from build123d import *

# Parameters (mm, degrees)
SKETCH3_W           = 5
SKETCH3_H           = 30
BOSS_EXTRUDE1_DEPTH = 5
SKETCH4_R           = 1.6
CUT_EXTRUDE1_DEPTH  = 75.540257579


with BuildPart() as part:
    # Sketch2 → Revolve1 (revolve)
    with BuildSketch(Plane.XY):
        with BuildLine():
            Line((0, 29), (0, 30))
            ThreePointArc((0, 30), (21.213203436, 21.213203436), (30, 0))
            Line((30, 0), (29, 0))
            ThreePointArc((29, 0), (20.506096654, 20.506096654), (0, 29))
        make_face()
    revolve(axis=Axis((0, 0, 0), (0, 1, 0)))

    # Sketch3 → Boss-Extrude1 (add)
    with BuildSketch(Plane.XZ):
        with Locations((0, -45)):
            Rectangle(SKETCH3_W, SKETCH3_H)
        with BuildLine():
            Line((-2.5, -38), (2.5, -38))
            Line((2.5, -38), (12.22277757, -26.308006594))
            Line((12.22277757, -26.308006594), (12.219091313, -26.300072385))
            ThreePointArc((12.219091313, -26.300072385), (-0.967100454, -29.109666297), (-13.937737405, -25.431073041))
            Line((-13.937737405, -25.431073041), (-14.41834904, -26.308006594))
            Line((-14.41834904, -26.308006594), (-2.5, -38))
        make_face()
    extrude(amount=-BOSS_EXTRUDE1_DEPTH)

    # Sketch4 → Cut-Extrude1 (cut, through all)
    with BuildSketch(Plane(origin=(2.5, 0, 0), x_dir=(0, 0, -1), z_dir=(1, 0, 0))):
        with Locations((55, 2.5)):
            Circle(SKETCH4_R)
    extrude(amount=-CUT_EXTRUDE1_DEPTH, mode=Mode.SUBTRACT)


solid = part.part
Could you check a few things on this model? Use its own coordinates, in mm. A direction names the side the tool comes from. Give positions to 0.01 mm unless a question says otherwise; leave off trailing zeros. Order: outer loops, then holes, each group sorted by start corner. A loop starts at its lowest first (then second) coordinate and runs counter-clockwise, first axis right, second up.
Item 1: If we section it at B-B, the plane y = 2.5: Write out the boundary of the cut face in (x, z).
Item 2: I'm going to push flat-ended pins straight in: pin 1 (4 mm diameter, centred on x = -4, y = 7.5, fed in from +Z); pin 2 (6 mm diameter, centred on x = 22.5, z = -24.5, fed in from +Y); pin 3 (10 mm diameter, centred on y = 23, z = 3, fed in from +X); pin 4 (1.5 mm diameter, centred on y = 3, z = -44, fed in from +X). Where does each tip first touch, or does it pass through?
Item 3: If we section it at C-C, the plane x = 9.5: Write out the boundary of the cut face in (y, z), plus the area to 3 significant figures.
Item 4: If we section it at A-A, the plane z = -55: Write out the boundary of the cut face in (x, y).
Item 5: If we section it at D-D, the plane y = 8: Write out the boundary of the cut face in (x, z), plus the area to 3 significant figures.
Item 6: If we mould it in two halves opening along Z, with no side actions, what happens to faces 3 (the face through (-8.543, 2.465, -32.072)), 4 (the face through (2.5, 2, -49)), 5 (the face through (0.035, 2.981, -56.526))? For each: pulls with the +Z half, pulls with the -Z half, needs draft (parallel to the pull), parting line crosses it, or undercut.
Item 7: For faces 1 (the face through (-2.5, 2, -49)), 2 (the face through (0, 2, -60)), which set-ups out of +Z, -Z, +X, -X, +Y, -Y let a thin tool reach every point of the face, with its end or its side?
Item 8: I need wall thicknesses on line 1 (Y direction, x = -1.3, z = -55); line 2 (X direction, y = 6.5, z = -25); line 3 (X direction, y = 16, z = 1). Which ranges of each line are inside material? Lowest first, please.
Values:
1. outline: (-14.42, -26.31) - (-2.5, -38) - (-2.5, -53.4) - (2.5, -53.4) - (2.5, -38) - (10.98, -27.81) arc R29.9 ccw (long way) to (-14.37, -26.22) - close; (-2.5, -60) - (2.5, -60) - (2.5, -56.6) - (-2.5, -56.6) - close; hole circle Ø57.78 at (0, 0)
2. pin 1: stops at z = 29.29
2. pin 2: passes through
2. pin 3: stops at x = 23.85
2. pin 4: stops at x = 2.5
3. outline: (0, -29.58) - (5, -29.58) - (5, -28.01) arc R28.46 ccw to (0, 28.46) - (0, 27.4) arc R27.4 cw to (0, -27.4) - close
3. area: 99.0 mm2
4. outline: (-2.5, 0) - (2.5, 0) - (2.5, 0.9) - (-2.5, 0.9) - close; (-2.5, 4.1) - (2.5, 4.1) - (2.5, 5) - (-2.5, 5) - close
5. outline: circle Ø57.83 at (0, 0); hole circle Ø55.75 at (0, 0)
5. area: 185 mm2
6. face 3: pulls with the -Z half
6. face 4: needs draft
6. face 5: undercut
7. face 1: -Z, -X, +Y, -Y
7. face 2: -Z, +X, -X, +Y, -Y
8. line 1: y = 0 to 0.9, 4.1 to 5
8. line 2: x = -15.26 to -13.18, 13.18 to 15.26
8. line 3: x = -25.36 to -24.17, 24.17 to 25.36
